```python
from build123d import *

# Parameters (mm, degrees)
Y_KSEKLIK_EKSTR_ZYON1_DEPTH = 110
IZIM2_R                     = 3
Y_KSEKLIK_EKSTR_ZYON2_DEPTH = 20
Y_KSEKLIK_EKSTR_ZYON3_DEPTH = 5
Y_KSEKLIK_EKSTR_ZYON4_START = 20
IZIM4_R                     = 3
Y_KSEKLIK_EKSTR_ZYON4_DEPTH = 20
Y_KSEKLIK_EKSTR_ZYON5_START = 5
Y_KSEKLIK_EKSTR_ZYON5_DEPTH = 5


with BuildPart() as part:
    # Çizim1 → Yükseklik-Ekstrüzyon1 (new body)
    with BuildSketch(Plane(origin=(0, 0, 0), x_dir=(1, 0, 0), z_dir=(0, 1, 0))):
        Polygon((4.041451884, 0), (2.020725942, 3.5), (-2.020725942, 3.5), (-4.041451884, 0), (-2.020725942, -3.5), (2.020725942, -3.5), align=None)
    extrude(amount=Y_KSEKLIK_EKSTR_ZYON1_DEPTH)

    # Çizim2 → Yükseklik-Ekstrüzyon2 (add)
    with BuildSketch(Plane(origin=(0, 110, 0), x_dir=(1, 0, 0), z_dir=(0, 1, 0))):
        with Locations(Location((0, 0, 0), (0, 0, 270))):
            Circle(IZIM2_R)
    extrude(amount=Y_KSEKLIK_EKSTR_ZYON2_DEPTH)

    # Çizim3 → Yükseklik-Ekstrüzyon3 (add)
    with BuildSketch(Plane(origin=(0, 130, 0), x_dir=(1, 0, 0), z_dir=(0, 1, 0))):
        with BuildLine():
            ThreePointArc((1.79891634, 2.08), (0, 2.75), (-1.79891634, 2.08))
            Line((-1.79891634, 2.08), (-1.79891634, -2.08))
            ThreePointArc((-1.79891634, -2.08), (0, -2.75), (1.79891634, -2.08))
            Line((1.79891634, -2.08), (1.79891634, 2.08))
        make_face()
    extrude(amount=Y_KSEKLIK_EKSTR_ZYON3_DEPTH)

    # Çizim4 → Yükseklik-Ekstrüzyon4 (add)
    with BuildSketch(Plane.XZ.offset(Y_KSEKLIK_EKSTR_ZYON4_START)):
        with Locations(Location((0, 0, 0), (0, 0, 90))):
            Circle(IZIM4_R)
    extrude(amount=-Y_KSEKLIK_EKSTR_ZYON4_DEPTH)

    # Çizim5 → Yükseklik-Ekstrüzyon5 (add)
    with BuildSketch(Plane.XZ.offset(20).offset(Y_KSEKLIK_EKSTR_ZYON5_START)):
        with BuildLine():
            ThreePointArc((1.79891634, 2.08), (0, 2.75), (-1.79891634, 2.08))
            Line((-1.79891634, 2.08), (-1.79891634, -2.08))
            ThreePointArc((-1.79891634, -2.08), (0, -2.75), (1.79891634, -2.08))
            Line((1.79891634, -2.08), (1.79891634, 2.08))
        make_face()
    extrude(amount=-Y_KSEKLIK_EKSTR_ZYON5_DEPTH)


solid = part.part
```
Input: part model. Units: mm. Frame: model coordinates. A direction names the side the tool comes from. Give positions to 0.01 mm unless a question says otherwise; leave off trailing zeros. Write each loop counter-clockwise with the first axis right and the second up, starting at its lowest first coordinate (ties: lowest second). Pieces come first, ordered by that corner, then holes. Notation, with made-up numbers: (24, 1) - (80, 1) arc R31 cw to (80, 34) - close; hole circle Ø2 at (-31.5, 9.5). An arc over 180 degrees is marked (long way). Write item = value, one per line. Start each with the question number.
1) Cut plane B-B (y = 78). Return loops of the section in (x, z).
2) Material intervals for L1, parallel to X at y = 71, z = -2.25; L2, parallel to Y at x = 2.5, z = -2.25; L3, parallel to X at y = 112.5, z = 0, sorted ascending. Write a range as [from, to].
3) Cut plane C-C (y = 121.5). Return loops of the section in (x, z), and give its area (3 significant figures).
4) Pin query (flat end, axial travel): pin 1 (1.5 mm diameter, centred on y = 48.5, z = 1.5, fed in from -X); pin 2 (1 mm diameter, centred on x = 2.5, y = -4.5, fed in from +Z); pin 3 (1.2 mm diameter, centred on y = 132, z = 0, fed in from -X). Return the tip coordinate at first contact, or that it passes through.
5) Cut plane A-A (x = 0). Return loops of the section in (y, z).
6) Reachability of faces 1 (the face through (1.799, -23, 0)), 2 (the face through (-1, 0, -3)), 3 (the face through (-1.799, 132, 0)), 4 (the face through (0.03, -22.54, 2.75)) from +Z, -Z, +X, -X, +Y, -Y: full face, straight path, thin tool, end or side. Return the list, or none.
Answers follow:
q1.outline = (-4.04, 0) - (-2.02, -3.5) - (2.02, -3.5) - (4.04, 0) - (2.02, 3.5) - (-2.02, 3.5) - close
q2.L1 = [-2.74, 2.74]
q2.L2 = [0, 110]
q2.L3 = [-3, 3]
q3.outline = circle Ø6 at (0, 0)
q3.area = 28.3 mm^2
q4.pin_1 = -3.61
q4.pin_2 = 2.24
q4.pin_3 = -1.8
q5.outline = (-25, -2.75) - (-20, -2.75) - (-20, -3) - (0, -3) - (0, -3.5) - (110, -3.5) - (110, -3) - (130, -3) - (130, -2.75) - (135, -2.75) - (135, 2.75) - (130, 2.75) - (130, 3) - (110, 3) - (110, 3.5) - (0, 3.5) - (0, 3) - (-20, 3) - (-20, 2.75) - (-25, 2.75) - close
q6.face_1 = +Z, -Z, +X, -Y
q6.face_2 = -Y
q6.face_3 = +Z, -Z, -X, +Y
q6.face_4 = +Z, -Y
